from build123d import *

# Parameters (mm, degrees)
F0_W     = 381
F0_H     = 304.8
F1_DEPTH = 25.4
F3_DEPTH = 25.4
F6_DEPTH = 25.401


with BuildPart() as f1:
    # F0 (on Top) → F1 (new body)
    with BuildSketch(Plane.XY):
        Rectangle(F0_W, F0_H)
    extrude(amount=F1_DEPTH)

    # F2 (on face) → F3 (cut)
    with BuildSketch(Plane.XY.offset(25.4)):
        Polygon((-190.5, 152.4), (-190.5, 61.934096), (-100.034096, 152.4), align=None)
        Polygon((0, -152.4), (-190.5, 61.934096), (-190.5, -152.4), align=None)
    extrude(amount=-F3_DEPTH, mode=Mode.SUBTRACT)

    # F4: F1 across plane


with BuildPart() as f1_1:
    add(f1.part)
    add(f1.part.mirror(Plane.YZ), mode=Mode.INTERSECT)

    # F5 (on face) → F6 (cut, through all)
    with BuildSketch(Plane.XY.offset(25.4)):
        Polygon((173.052639, 61.420945), (100.330883, 134.142701), (99.771466, 41.838474), (121.261792, 3.15037), align=None)
    extrude(amount=-F6_DEPTH, mode=Mode.SUBTRACT)


solid = f1_1.part
Could you check a few things on this model? Use its own coordinates, in mm. A direction names the side the tool comes from. Give positions to 0.01 mm unless a question says otherwise; leave off trailing zeros. Order: outer loops, then holes, each group sorted by start corner. A loop starts at its lowest first (then second) coordinate and runs counter-clockwise, first axis right, second up.
Item 1: If we section it at A-A, the plane y = 73: Write out the boundary of the cut face in (x, z), plus the area to 3 significant figures.
Item 2: If we section it at D-D, the plane x = -148.5: Write out the boundary of the cut face in (y, z).
Item 3: If we section it at C-C, the plane x = 133: Write out the boundary of the cut face in (y, z), plus the area to 3 significant figures.
Item 4: If we mould it in two halves opening along Y, with no side actions, what happens to faces 1 (the face through (137.201, 97.273, 12.878)), 2 (the face through (-1, 152.4, 13)), 3 (the face through (-3, 36, 25.4))? For each: pulls with the +Y half, pulls with the -Y half, needs draft (parallel to the pull), parting line crosses it, or undercut.
Item 5: For faces 4 (the face through (145.9, 106.534, 12.878)), 5 (the face through (110.366, 22.765, 12.878)), which set-ups out of +Z, -Z, +X, -X, +Y, -Y let a thin tool reach every point of the face, with its end or its side?
Item 6: I need wall thicknesses on line 1 (Y direction, x = 108, z = 8) (3 decimals); line 2 (X direction, y = 130, z = 8.25); line 3 (X direction, y = 26, z = 6.25). Which ranges of each line are inside material? Lowest first, please.
Item 7: If we section it at B-B, the plane z = 15: Write out the boundary of the cut face in (x, y), plus the area to 3 significant figures.
Item 8: I'm going to push flat-ended pins straight in: pin 1 (3 mm diameter, centred on y = -89, z = 18.5, fed in from +X); pin 2 (5 mm diameter, centred on y = -67.5, z = 8.5, fed in from -X); pin 3 (2 mm diameter, centred on y = 91, z = 20, fed in from +X). Where does each tip first touch, or does it pass through?
Values:
1. outline: (-179.43, 0) - (99.96, 0) - (99.96, 25.4) - (-179.43, 25.4) - close; (161.47, 0) - (179.43, 0) - (179.43, 25.4) - (161.47, 25.4) - close
1. area: 7,550 mm2
2. outline: (14.68, 0) - (103.93, 0) - (103.93, 25.4) - (14.68, 25.4) - close
3. outline: (-2.76, 0) - (16.36, 0) - (16.36, 25.4) - (-2.76, 25.4) - close; (101.47, 0) - (119.43, 0) - (119.43, 25.4) - (101.47, 25.4) - close
3. area: 942 mm2
4. face 1: undercut
4. face 2: pulls with the +Y half
4. face 3: needs draft
5. face 4: +Z, -Z, +X, +Y
5. face 5: +Z, -Z
6. line 1: y = -30.888 to 27.025, 126.474 to 144.434
6. line 2: x = -122.43 to 100.31, 104.47 to 122.43
6. line 3: x = -158.56 to 108.57, 141.57 to 158.56
7. outline: (-190.5, 61.93) - (0, -152.4) - (190.5, 61.93) - (100.03, 152.4) - (-100.03, 152.4) - close; hole (99.77, 41.84) - (121.26, 3.15) - (173.05, 61.42) - (100.33, 134.14) - close
7. area: 62,100 mm2
8. pin 1: stops at x = 57.68
8. pin 2: stops at x = -77.68
8. pin 3: stops at x = 162.43
